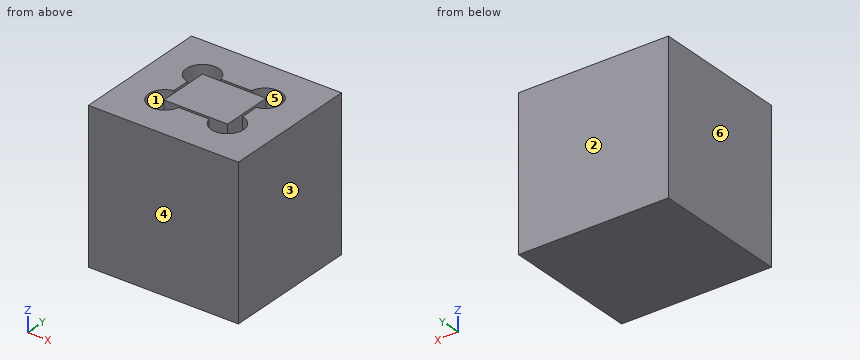
```python
from build123d import *

# Parameters (mm, degrees)
ESQUISSE1_W             = 12
ESQUISSE1_H             = 11
EXTRUSION1_DEPTH        = 12
ENL_V_MAT_EXTRU_1_DEPTH = 2.5
ESQUISSE3_W             = 5.1
ESQUISSE3_H             = 4.1
EXTRUSION2_DEPTH        = 2.5


with BuildPart() as part:
    # Esquisse1 → Extrusion1 (new body)
    with BuildSketch(Plane.XY):
        with Locations((6, 5.5)):
            Rectangle(ESQUISSE1_W, ESQUISSE1_H)
    extrude(amount=EXTRUSION1_DEPTH)

    # Esquisse2 → Enlèv. mat.-Extru.1 (cut)
    with BuildSketch(Plane.XY.offset(12)):
        with BuildLine():
            Line((4.775735082, 7.75), (7.224264918, 7.75))
            ThreePointArc((7.224264918, 7.75), (9.419238816, 8.419238816), (8.75, 6.224264918))
            Line((8.75, 6.224264918), (8.75, 4.775735082))
            ThreePointArc((8.75, 4.775735082), (9.419238816, 2.580761184), (7.224264918, 3.25))
            Line((7.224264918, 3.25), (4.775735082, 3.25))
            ThreePointArc((4.775735082, 3.25), (2.580761184, 2.580761184), (3.25, 4.775735082))
            Line((3.25, 4.775735082), (3.25, 6.224264918))
            ThreePointArc((3.25, 6.224264918), (2.580761184, 8.419238816), (4.775735082, 7.75))
        make_face()
    extrude(amount=-ENL_V_MAT_EXTRU_1_DEPTH, mode=Mode.SUBTRACT)

    # Esquisse3 → Extrusion2 (add)
    with BuildSketch(Plane.XY.offset(9.5)):
        with Locations((6, 5.5)):
            Rectangle(ESQUISSE3_W, ESQUISSE3_H)
    extrude(amount=EXTRUSION2_DEPTH)


solid = part.part
```
For this review, take the finished solid that the model builds, in its own axes (mm). Face numbers are marked on the shaded views. A direction names the side the tool comes from. Coordinates: 2 decimals unless noted, no trailing zeros. Loops run counter-clockwise (first coordinate to the right, second up) from the corner with the lowest first, then second, coordinate; pieces in that order, holes last. Notation, with made-up numbers: (-26, -27) - (5, -27) arc R9 ccw to (5, -16) - close; hole circle Ø11 at (-12, -12.5). An arc over 180 degrees is marked (long way). Use one line per item in the form item = value. Start each with the question number.
1) To check wall thickness, follow probe 1 along X at (y, z) = (3.5, 10.5); probe 2 along Y at (x, z) = (3.5, 10.4); probe 3 along X at (y, z) = (5.75, 11.75). State the ranges of each line that lie inside material, in increasing order. Write a range as from..to.
2) For the marked faces 1 and 2, list the 3-axis set-ups (+Z, -Z, +X, -X, +Y, -Y) from which the entire face can be reached by the end or side of a thin tool; tool diameter is ignored.
3) For pin 1 (1.6 mm diameter, centred on y = 5.5, z = 11.5, fed in from -X), flat-tipped, find the tip position at first contact; note if it passes through.
4) Draft analysis for pull direction X (two halves, no side actions). For the marked faces 3, 4, 5 and 6, state which applies: released by +X, released by -X, zero draft, split by the parting line, or undercut.
5) Take a section at B-B (x = 9.25). State the section outline as (y, z) points.
6) Take a section at A-A (y = 4). State the section outline as (x, z) points, plus the area to 3 significant figures.
From the geometry:
q1.probe_1 = 0..2.2, 3.45..8.55, 9.8..12
q1.probe_2 = 0..2.2, 3.45..7.55, 8.8..11
q1.probe_3 = 0..3.25, 3.45..8.55, 8.75..12
q2.face_1 = +Z
q2.face_2 = +Z, -Z, +X, -X, +Y
q3.pin_1 = 0
q4.face_3 = released by +X
q4.face_4 = zero draft
q4.face_5 = undercut
q4.face_6 = released by -X
q5.outline = (0, 0) - (11, 0) - (11, 12) - (8.56, 12) - (8.56, 9.5) - (6.44, 9.5) - (6.44, 12) - (4.56, 12) - (4.56, 9.5) - (2.44, 9.5) - (2.44, 12) - (0, 12) - close
q6.outline = (0, 0) - (12, 0) - (12, 12) - (9.7, 12) - (9.7, 9.5) - (8.55, 9.5) - (8.55, 12) - (3.45, 12) - (3.45, 9.5) - (2.3, 9.5) - (2.3, 12) - (0, 12) - close
q6.area = 138 mm2
